```python
from build123d import *

# Parameters (mm, degrees)
F0_W      = 90
F0_H      = 80
F0_R      = 5
F0_R_2    = 2.25
F1_DEPTH  = 5
F2_DEPTH  = 10
F3_W      = 8
F3_H      = 8
F3_H_2    = 6
F4_DEPTH  = 10.001
F5_R      = 2.25
F6_DEPTH  = 20
F7_R      = 2.25
F8_DEPTH  = 20
F9_R      = 2.25
F10_DEPTH = 10.001


# Not quite as in the source:
# - a feature names something its author has since deleted; it is built from what else it names


with BuildPart() as f1:
    # F0 (on Front) → F1 (new body)
    with BuildSketch(Plane.XZ):
        with Locations((45, 40)):
            Rectangle(F0_W, F0_H)
        Polygon((40, 23), (40, 17), (6, 17), (6, 23), (6, 41), (6, 47), (40, 47), (40, 41), align=None, mode=Mode.SUBTRACT)
        Polygon((84, 23), (84, 17), (50, 17), (50, 23), (50, 41), (50, 47), (84, 47), (84, 41), align=None, mode=Mode.SUBTRACT)
        Polygon((6, 73), (6, 79), (40, 79), (40, 73), (40, 55), (40, 49), (6, 49), (6, 55), align=None, mode=Mode.SUBTRACT)
        Polygon((84, 55), (84, 49), (50, 49), (50, 55), (50, 73), (50, 79), (84, 79), (84, 73), align=None, mode=Mode.SUBTRACT)
        Polygon((40, 79), (6, 79), (6, 73), (6, 55), (6, 49), (40, 49), (40, 55), (40, 73), align=None)
        with BuildLine():
            ThreePointArc((16, 55), (11, 50), (6, 55))
            ThreePointArc((6, 55), (11, 60), (16, 55))
        make_face(mode=Mode.SUBTRACT)
        with Locations((35, 55)):
            Circle(F0_R, mode=Mode.SUBTRACT)
        with BuildLine():
            ThreePointArc((16, 73), (11, 68), (6, 73))
            ThreePointArc((6, 73), (11, 78), (16, 73))
        make_face(mode=Mode.SUBTRACT)
        with Locations((35, 73)):
            Circle(F0_R, mode=Mode.SUBTRACT)
        Polygon((50, 49), (84, 49), (84, 55), (84, 73), (84, 79), (50, 79), (50, 73), (50, 55), align=None)
        with BuildLine():
            ThreePointArc((60, 55), (55, 50), (50, 55))
            ThreePointArc((50, 55), (55, 60), (60, 55))
        make_face(mode=Mode.SUBTRACT)
        with Locations((79, 55)):
            Circle(F0_R, mode=Mode.SUBTRACT)
        with BuildLine():
            ThreePointArc((60, 73), (55, 68), (50, 73))
            ThreePointArc((50, 73), (55, 78), (60, 73))
        make_face(mode=Mode.SUBTRACT)
        with Locations((79, 73)):
            Circle(F0_R, mode=Mode.SUBTRACT)
        Polygon((6, 17), (40, 17), (40, 23), (40, 41), (40, 47), (6, 47), (6, 41), (6, 23), align=None)
        with BuildLine():
            ThreePointArc((16, 23), (11, 18), (6, 23))
            ThreePointArc((6, 23), (11, 28), (16, 23))
        make_face(mode=Mode.SUBTRACT)
        with Locations((35, 23)):
            Circle(F0_R, mode=Mode.SUBTRACT)
        with BuildLine():
            ThreePointArc((16, 41), (11, 36), (6, 41))
            ThreePointArc((6, 41), (11, 46), (16, 41))
        make_face(mode=Mode.SUBTRACT)
        with Locations((35, 41)):
            Circle(F0_R, mode=Mode.SUBTRACT)
        Polygon((50, 17), (84, 17), (84, 23), (84, 41), (84, 47), (50, 47), (50, 41), (50, 23), align=None)
        with BuildLine():
            ThreePointArc((60, 23), (55, 18), (50, 23))
            ThreePointArc((50, 23), (55, 28), (60, 23))
        make_face(mode=Mode.SUBTRACT)
        with Locations((79, 23)):
            Circle(F0_R, mode=Mode.SUBTRACT)
        with BuildLine():
            ThreePointArc((60, 41), (55, 36), (50, 41))
            ThreePointArc((50, 41), (55, 46), (60, 41))
        make_face(mode=Mode.SUBTRACT)
        with Locations((79, 41)):
            Circle(F0_R, mode=Mode.SUBTRACT)
        with Locations((79, 41)):
            Circle(F0_R)
        with Locations((79, 41)):
            Circle(F0_R_2, mode=Mode.SUBTRACT)
        with BuildLine():
            ThreePointArc((16, 23), (11, 28), (6, 23))
            ThreePointArc((6, 23), (11, 18), (16, 23))
        make_face()
        with Locations((11, 23)):
            Circle(F0_R_2, mode=Mode.SUBTRACT)
        with BuildLine():
            ThreePointArc((16, 73), (11, 78), (6, 73))
            ThreePointArc((6, 73), (11, 68), (16, 73))
        make_face()
        with Locations((11, 73)):
            Circle(F0_R_2, mode=Mode.SUBTRACT)
        with Locations((35, 73)):
            Circle(F0_R)
        with Locations((35, 73)):
            Circle(F0_R_2, mode=Mode.SUBTRACT)
        with BuildLine():
            ThreePointArc((60, 73), (55, 78), (50, 73))
            ThreePointArc((50, 73), (55, 68), (60, 73))
        make_face()
        with Locations((55, 73)):
            Circle(F0_R_2, mode=Mode.SUBTRACT)
        with Locations((79, 73)):
            Circle(F0_R)
        with Locations((79, 73)):
            Circle(F0_R_2, mode=Mode.SUBTRACT)
        with Locations((79, 55)):
            Circle(F0_R)
        with Locations((79, 55)):
            Circle(F0_R_2, mode=Mode.SUBTRACT)
        with BuildLine():
            ThreePointArc((60, 55), (55, 60), (50, 55))
            ThreePointArc((50, 55), (55, 50), (60, 55))
        make_face()
        with Locations((55, 55)):
            Circle(F0_R_2, mode=Mode.SUBTRACT)
        with Locations((35, 55)):
            Circle(F0_R)
        with Locations((35, 55)):
            Circle(F0_R_2, mode=Mode.SUBTRACT)
        with BuildLine():
            ThreePointArc((16, 55), (11, 60), (6, 55))
            ThreePointArc((6, 55), (11, 50), (16, 55))
        make_face()
        with Locations((11, 55)):
            Circle(F0_R_2, mode=Mode.SUBTRACT)
        with Locations((35, 41)):
            Circle(F0_R)
        with Locations((35, 41)):
            Circle(F0_R_2, mode=Mode.SUBTRACT)
        with Locations((35, 23)):
            Circle(F0_R)
        with Locations((35, 23)):
            Circle(F0_R_2, mode=Mode.SUBTRACT)
        with BuildLine():
            ThreePointArc((16, 41), (11, 46), (6, 41))
            ThreePointArc((6, 41), (11, 36), (16, 41))
        make_face()
        with Locations((11, 41)):
            Circle(F0_R_2, mode=Mode.SUBTRACT)
        with BuildLine():
            ThreePointArc((60, 23), (55, 28), (50, 23))
            ThreePointArc((50, 23), (55, 18), (60, 23))
        make_face()
        with Locations((55, 23)):
            Circle(F0_R_2, mode=Mode.SUBTRACT)
        with BuildLine():
            ThreePointArc((60, 41), (55, 46), (50, 41))
            ThreePointArc((50, 41), (55, 36), (60, 41))
        make_face()
        with Locations((55, 41)):
            Circle(F0_R_2, mode=Mode.SUBTRACT)
        with Locations((79, 23)):
            Circle(F0_R)
        with Locations((79, 23)):
            Circle(F0_R_2, mode=Mode.SUBTRACT)
    extrude(amount=F1_DEPTH)

    # F0 (on Front) → F2 (join)
    with BuildSketch(Plane.XZ):
        with Locations((45, 40)):
            Rectangle(F0_W, F0_H)
        Polygon((40, 23), (40, 17), (6, 17), (6, 23), (6, 41), (6, 47), (40, 47), (40, 41), align=None, mode=Mode.SUBTRACT)
        Polygon((84, 23), (84, 17), (50, 17), (50, 23), (50, 41), (50, 47), (84, 47), (84, 41), align=None, mode=Mode.SUBTRACT)
        Polygon((6, 73), (6, 79), (40, 79), (40, 73), (40, 55), (40, 49), (6, 49), (6, 55), align=None, mode=Mode.SUBTRACT)
        Polygon((84, 55), (84, 49), (50, 49), (50, 55), (50, 73), (50, 79), (84, 79), (84, 73), align=None, mode=Mode.SUBTRACT)
        Polygon((50, 49), (84, 49), (84, 55), (84, 73), (84, 79), (50, 79), (50, 73), (50, 55), align=None)
        with BuildLine():
            ThreePointArc((60, 55), (55, 50), (50, 55))
            ThreePointArc((50, 55), (55, 60), (60, 55))
        make_face(mode=Mode.SUBTRACT)
        with Locations((79, 55)):
            Circle(F0_R, mode=Mode.SUBTRACT)
        with BuildLine():
            ThreePointArc((60, 73), (55, 68), (50, 73))
            ThreePointArc((50, 73), (55, 78), (60, 73))
        make_face(mode=Mode.SUBTRACT)
        with Locations((79, 73)):
            Circle(F0_R, mode=Mode.SUBTRACT)
        Polygon((50, 17), (84, 17), (84, 23), (84, 41), (84, 47), (50, 47), (50, 41), (50, 23), align=None)
        with BuildLine():
            ThreePointArc((60, 23), (55, 18), (50, 23))
            ThreePointArc((50, 23), (55, 28), (60, 23))
        make_face(mode=Mode.SUBTRACT)
        with Locations((79, 23)):
            Circle(F0_R, mode=Mode.SUBTRACT)
        with BuildLine():
            ThreePointArc((60, 41), (55, 36), (50, 41))
            ThreePointArc((50, 41), (55, 46), (60, 41))
        make_face(mode=Mode.SUBTRACT)
        with Locations((79, 41)):
            Circle(F0_R, mode=Mode.SUBTRACT)
        Polygon((6, 17), (40, 17), (40, 23), (40, 41), (40, 47), (6, 47), (6, 41), (6, 23), align=None)
        with BuildLine():
            ThreePointArc((16, 23), (11, 18), (6, 23))
            ThreePointArc((6, 23), (11, 28), (16, 23))
        make_face(mode=Mode.SUBTRACT)
        with Locations((35, 23)):
            Circle(F0_R, mode=Mode.SUBTRACT)
        with BuildLine():
            ThreePointArc((16, 41), (11, 36), (6, 41))
            ThreePointArc((6, 41), (11, 46), (16, 41))
        make_face(mode=Mode.SUBTRACT)
        with Locations((35, 41)):
            Circle(F0_R, mode=Mode.SUBTRACT)
        Polygon((40, 79), (6, 79), (6, 73), (6, 55), (6, 49), (40, 49), (40, 55), (40, 73), align=None)
        with BuildLine():
            ThreePointArc((16, 55), (11, 50), (6, 55))
            ThreePointArc((6, 55), (11, 60), (16, 55))
        make_face(mode=Mode.SUBTRACT)
        with Locations((35, 55)):
            Circle(F0_R, mode=Mode.SUBTRACT)
        with BuildLine():
            ThreePointArc((16, 73), (11, 68), (6, 73))
            ThreePointArc((6, 73), (11, 78), (16, 73))
        make_face(mode=Mode.SUBTRACT)
        with Locations((35, 73)):
            Circle(F0_R, mode=Mode.SUBTRACT)
    extrude(amount=F2_DEPTH)

    # F3 (on face) → F4 (cut, through all)
    with BuildSketch(Plane.XZ.offset(10)):
        with Locations((45, 64)):
            Rectangle(F3_W, F3_H)
        with Locations((45, 77)):
            Rectangle(F3_W, F3_H_2)
        with Locations((45, 16)):
            Rectangle(F3_W, F3_H)
        with Locations((45, 3)):
            Rectangle(F3_W, F3_H_2)
    extrude(amount=-F4_DEPTH, mode=Mode.SUBTRACT)

    # F5 (on face) → F6 (cut)
    with BuildSketch(Plane.XY.offset(80)):
        with Locations((45, -5)):
            Circle(F5_R)
    extrude(amount=-F6_DEPTH, mode=Mode.SUBTRACT)

    # F7 (on face) → F8 (cut)
    with BuildSketch(Plane(origin=(0, 0, 0), x_dir=(1, 0, 0), z_dir=(0, 0, -1))):
        with Locations((45, 5)):
            Circle(F7_R)
    extrude(amount=-F8_DEPTH, mode=Mode.SUBTRACT)

    # F9 (on face) → F10 (cut, through all)
    with BuildSketch(Plane.XZ.offset(10)):
        with Locations((45, 33)):
            Circle(F9_R)
        with Locations((12, 5.5)):
            Circle(F9_R)
        with Locations((78, 5.5)):
            Circle(F9_R)
    extrude(amount=-F10_DEPTH, mode=Mode.SUBTRACT)


solid = f1.part
```
Work out the finished part from the listing and answer in its coordinate system (mm). A direction names the side the tool comes from. Coordinates: 2 decimals unless noted, no trailing zeros. Loops run counter-clockwise (first coordinate to the right, second up) from the corner with the lowest first, then second, coordinate; pieces in that order, holes last. Notation, with made-up numbers: (-17, 22.25) - (15, 22.25) arc R23 ccw to (15, 46.25) - close; hole circle Ø10 at (-39.75, 47.25). An arc over 180 degrees is marked (long way). Use a Markdown table: item, result.
Item 1: Find section B-B, the plane z = 73. State how many separate pieces and enclosed holes the cut face has, and give its area (3 significant figures).
Evaluation:
| item | result |
|---|---|
| separate pieces | 5 |
| enclosed holes | 1 |
| area | 594 mm2 |
Item 2: Consider probe 1 along Z at (x, y) = (55, -2.35); probe 2 along Z at (x, y) = (35, -7.5); probe 3 along X at (y, z) = (-2, 61). Determine where each line is inside the solid, lowest interval first. Write a range as from..to.
Evaluation:
| item | result |
|---|---|
| probe 1 | z = 0..20.75, 25.25..38.75, 43.25..52.75, 57.25..70.75, 75.25..80 |
| probe 2 | z = 0..18, 28..36, 46..50, 60..68, 78..80 |
| probe 3 | x = 0..41, 49..90 |
Item 3: Find section C-C, the plane z = 11. Determine the outline of the cut face in (x, y).
Evaluation:
| item | result |
|---|---|
| outline | (0, -10) - (90, -10) - (90, 0) - (0, 0) - close; hole circle Ø4.5 at (45, -5) |
Item 4: The mould has two halves that part along X. Classify faces 1 (the flat face through (36, -5, 38.8)), 2 (the flat face through (0, -5, 39)), 3 (the flat face through (90, -5, 39)): +X half, -X half, draft (parallel to the pull), parting line (faces both ways), or undercut.
Evaluation:
| item | result |
|---|---|
| face 1 | undercut |
| face 2 | -X half |
| face 3 | +X half |
Item 5: Given pin 1 Ø4 at (x, y) = (45, -5) entering from +Z; pin 2 Ø5 at (x, z) = (79, 23) entering from -Y, each flat-ended and moving along its own axis, determine where each tip first touches the part or whether it passes through.
Evaluation:
| item | result |
|---|---|
| pin 1 | stops at z = 60 |
| pin 2 | stops at y = -5 |
Item 6: For faces 4 (the cylindrical face through (8, -7, 59)), 5 (the flat face through (49, -5, 64)), 6 (the flat face through (41, -5, 3)), determine the directions among +Z, -Z, +X, -X, +Y, -Y from which every point of the face is accessible in a straight line to the end or side of a thin tool.
Evaluation:
| item | result |
|---|---|
| face 4 | -Y |
| face 5 | +Y, -Y |
| face 6 | -Z, +Y, -Y |
Item 7: Find section A-A, the plane z = 33. Determine the outline of the cut face in (x, y).
Evaluation:
| item | result |
|---|---|
| outline | (0, -10) - (42.75, -10) - (42.75, 0) - (0, 0) - close; (47.25, -10) - (90, -10) - (90, 0) - (47.25, 0) - close |
